Verification items for this drawing (mm, ordinates from the low corner). A direction names the side the tool comes from. Round coordinates to 2 decimals unless told otherwise and drop trailing zeros. Write each loop counter-clockwise with the first axis right and the second up, starting at its lowest first coordinate (ties: lowest second). Pieces come first, ordered by that corner, then holes. Notation, with made-up numbers: (69, 3.5) -> (117, 3.5) arc R33 cw to (117, 36.5) -> close; hole circle Ø7 at (30, 82.25). An arc over 180 degrees is marked (long way). Return JSON: item names as keys, results as strings. Group by question number.
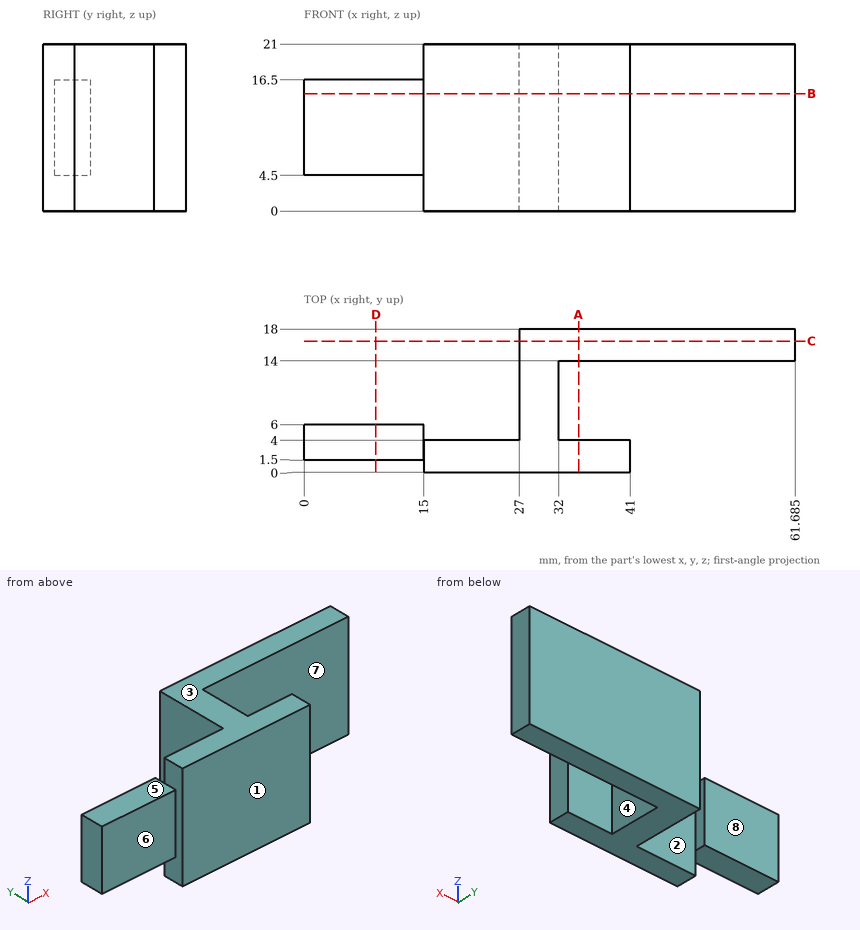
1) Sectioned sample at B-B on z = 14.75. Enter the section's corners in (x, y) (1 decimal).
2) Sectioned sample at D-D on x = 9. Enter the section's corners in (y, z).
3) Sectioned sample at C-C on y = 16.5. Enter the section's corners in (x, z) (1 decimal).
4) Material ranges on probe 1 along Y at (x, z) = (35, 19); probe 2 along X at (y, z) = (10.5, 20); probe 3 along Y at (x, z) = (58, 5.5), recorded low to high. Write a range as [from, to].
5) Go/stop test with flat-tipped pins: P1, Ø9.5, axis at x = 20.5, z = 10, coming from the +Y side; P2, Ø5, axis at x = 10, y = 4, coming from the +Z side; P3, Ø9.5, axis at x = 4.5, z = 10.5, coming from the +Y side. Record where each tip stops, or that it passes through.
6) Sectioned sample at A-A on x = 34.5. Enter the section's corners in (y, z).
7) Mould release check, pull along Y, two halves, no side actions. Record for the marked faces 1, 2, 3 and 4: +Y half, -Y half, draft (parallel to the pull), parting line (faces both ways), or undercut.
8) Tool access check on the marked faces 5, 6, 7 and 8. Record the directions out of +Z, -Z, +X, -X, +Y, -Y that give a thin tool (end or side, any length) a straight path to the whole face; none if there is none.
Evaluation:
{
 "1": {"outline": "(0, 1.5) -> (15, 1.5) -> (15, 0) -> (41, 0) -> (41, 4) -> (32, 4) -> (32, 14) -> (61.7, 14) -> (61.7, 18) -> (27, 18) -> (27, 4) -> (15, 4) -> (15, 6) -> (0, 6) -> close"},
 "2": {"outline": "(1.5, 4.5) -> (6, 4.5) -> (6, 16.5) -> (1.5, 16.5) -> close"},
 "3": {"outline": "(27, 0) -> (61.7, 0) -> (61.7, 21) -> (27, 21) -> close"},
 "4": {"probe 1": "y = [0, 4], [14, 18]", "probe 2": "x = [27, 32]", "probe 3": "y = [14, 18]"},
 "5": {"P1": "stops at y = 4", "P2": "stops at z = 16.5", "P3": "stops at y = 6"},
 "6": {"outline": "(0, 0) -> (4, 0) -> (4, 21) -> (0, 21) -> close; (14, 0) -> (18, 0) -> (18, 21) -> (14, 21) -> close"},
 "7": {"face 1": "-Y half", "face 2": "+Y half", "face 3": "draft", "face 4": "undercut"},
 "8": {"face 5": "+Z, -X, +Y, -Y", "face 6": "+Z, -Z, -X, -Y", "face 7": "+Z, -Z, +X", "face 8": "+Z, -Z, -X, +Y"}
}
